```python
from build123d import *

# Parameters (mm, degrees)
EXTRUDE_1_DEPTH     = 3
CUT_EXTRUDE_3_DEPTH = 3


with BuildPart() as part:
    # 草图1 → 凸台-拉伸1 (new body)
    with BuildSketch(Plane(origin=(0, 0, 0), x_dir=(1, 0, 0), z_dir=(0, 1, 0))):
        with BuildLine():
            Line((-184.615743852, 100), (185.384256148, 100))
            ThreePointArc((185.384256148, 100), (195.990857866, 95.606601718), (200.384256148, 85))
            Line((200.384256148, 85), (200.384256148, -85))
            ThreePointArc((200.384256148, -85), (195.990857866, -95.606601718), (185.384256148, -100))
            Line((185.384256148, -100), (-184.615743852, -100))
            ThreePointArc((-184.615743852, -100), (-195.22234557, -95.606601718), (-199.615743852, -85))
            Line((-199.615743852, -85), (-199.615743852, 85))
            ThreePointArc((-199.615743852, 85), (-195.22234557, 95.606601718), (-184.615743852, 100))
        make_face()
    extrude(amount=EXTRUDE_1_DEPTH)

    # 草图2 → 切除-拉伸3 (cut)
    with BuildSketch(Plane(origin=(0, 3, 0), x_dir=(1, 0, 0), z_dir=(0, 1, 0))):
        with BuildLine():
            Line((-175, 70), (-25, 70))
            ThreePointArc((-25, 70), (-15, 60), (-25, 50))
            Line((-25, 50), (-175, 50))
            ThreePointArc((-175, 50), (-185, 60), (-175, 70))
        make_face()
        with BuildLine():
            Line((25, 50), (175, 50))
            ThreePointArc((175, 50), (185, 60), (175, 70))
            Line((175, 70), (25, 70))
            ThreePointArc((25, 70), (15, 60), (25, 50))
        make_face()
    extrude(amount=-CUT_EXTRUDE_3_DEPTH, mode=Mode.SUBTRACT)


solid = part.part
```
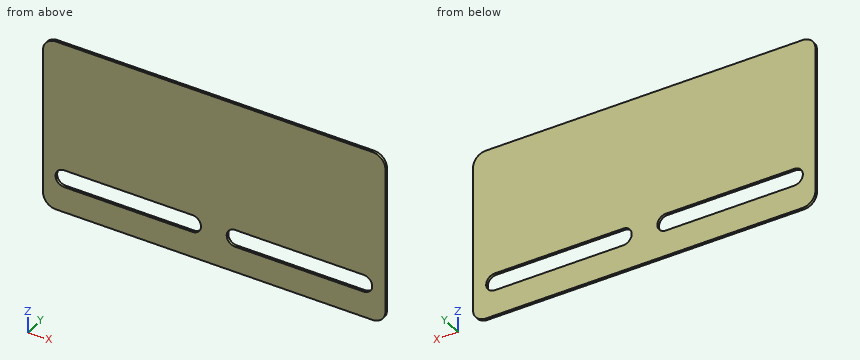
Source: CAD feature listing. Evaluate the final solid. Frame: model axes, mm. Round coordinates to 2 decimals unless told otherwise and drop trailing zeros. Loops run counter-clockwise (first coordinate to the right, second up) from the corner with the lowest first, then second, coordinate; pieces in that order, holes last.
(1) Section query B-B (y = 1.4). Output: boundary loops of the cut face in (x, z), and give its area (3 significant figures).
From the geometry:
outline: (-199.62, -85) arc R15 ccw to (-184.62, -100) - (185.38, -100) arc R15 ccw to (200.38, -85) - (200.38, 85) arc R15 ccw to (185.38, 100) - (-184.62, 100) arc R15 ccw to (-199.62, 85) - close; hole (-175, -70) - (-25, -70) arc R10 ccw to (-25, -50) - (-175, -50) arc R10 ccw to start; hole (25, -70) - (175, -70) arc R10 ccw to (175, -50) - (25, -50) arc R10 ccw to start
area: 73,200 mm2
(2) Section query A-A (x = 56). Output: boundary loops of the cut face in (y, z), and give its area (3 significant figures).
From the geometry:
outline: (0, -100) - (3, -100) - (3, -70) - (0, -70) - close; (0, -50) - (3, -50) - (3, 100) - (0, 100) - close
area: 540 mm2
(3) Section query C-C (z = -60). Output: boundary loops of the cut face in (x, y).
From the geometry:
outline: (-199.62, 0) - (-185, 0) - (-185, 3) - (-199.62, 3) - close; (-15, 0) - (15, 0) - (15, 3) - (-15, 3) - close; (185, 0) - (200.38, 0) - (200.38, 3) - (185, 3) - close
(4) Material intervals for probe 1 along Z at (x, y) = (141.5, 0.35), sorted ascending.
From the geometry:
probe 1: z = -100 to -70, -50 to 100
